```python
from build123d import *

# Parameters (mm, degrees)
SKETCH_1_R             = 120
EXTRUDE_1_DEPTH        = 20
SKETCH_2_R             = 100
EXTRUDE_2_DEPTH        = 50
SKETCH_3_R             = 8.5
CUT_EXTRUDE_1_DEPTH    = 80
SKETCH_4_R             = 20
EXTRUDE_3_DEPTH        = 20
HOLE_WIZARD_M161_D     = 14
HOLE_WIZARD_M161_DEPTH = 20
HOLE_WIZARD_M161_TIP   = 4.206024333
CHAMFER_1_SIZE         = 3
CHAMFER_2_SIZE         = 3


with BuildPart() as part:
    # Эскиз1 → Бобышка-Вытянуть1 (new body)
    with BuildSketch(Plane(origin=(0, 0, 0), x_dir=(1, 0, 0), z_dir=(0, 1, 0))):
        Circle(SKETCH_1_R)
    extrude(amount=EXTRUDE_1_DEPTH)

    # Эскиз2 → Бобышка-Вытянуть2 (add)
    with BuildSketch(Plane(origin=(0, 20, 0), x_dir=(1, 0, 0), z_dir=(0, 1, 0))):
        Circle(SKETCH_2_R)
    extrude(amount=EXTRUDE_2_DEPTH)

    # Эскиз3 → Вырез-Вытянуть1 (cut)
    with BuildSketch(Plane(origin=(0, 70, 0), x_dir=(1, 0, 0), z_dir=(0, 1, 0))):
        with Locations((0, 60)):
            Circle(SKETCH_3_R)
        with Locations((60, 0)):
            Circle(SKETCH_3_R)
        with Locations((0, -60)):
            Circle(SKETCH_3_R)
        with Locations((-60, 0)):
            Circle(SKETCH_3_R)
    extrude(amount=-CUT_EXTRUDE_1_DEPTH, mode=Mode.SUBTRACT)

    # Эскиз4 → Бобышка-Вытянуть3 (add)
    with BuildSketch(Plane.XZ):
        Circle(SKETCH_4_R)
    extrude(amount=EXTRUDE_3_DEPTH)

    # Отверстие обработанное метчиком M161
    with Locations(Plane(origin=(0, 70, 0), x_dir=(1, 0, 0), z_dir=(0, 1, 0))):
        with Locations((0, 0)):
            Hole(HOLE_WIZARD_M161_D / 2, depth=HOLE_WIZARD_M161_DEPTH)
            with Locations((0, 0, -(HOLE_WIZARD_M161_DEPTH + HOLE_WIZARD_M161_TIP / 2))):  # 118° drill point
                Cone(0, HOLE_WIZARD_M161_D / 2, HOLE_WIZARD_M161_TIP, mode=Mode.SUBTRACT)

    # Фаска1
    chamfer_1_edges = [part.edges().sort_by_distance(p)[0] for p in [
        (-120, 0, 0),
        (-120, 20, 0),
        (-100, 70, 0),
    ]]
    chamfer(chamfer_1_edges, length=CHAMFER_1_SIZE)

    # Фаска2
    chamfer_2_edges = [part.edges().sort_by_distance(p)[0] for p in [
        (-20, -20, 0),
    ]]
    chamfer(chamfer_2_edges, length=CHAMFER_2_SIZE)


solid = part.part
```
Source: CAD feature listing. Evaluate the final solid. Frame: model axes, mm. A direction names the side the tool comes from. Round coordinates to 2 decimals unless told otherwise and drop trailing zeros. Write each loop counter-clockwise with the first axis right and the second up, starting at its lowest first coordinate (ties: lowest second). Pieces come first, ordered by that corner, then holes. Notation, with made-up numbers: M 52,9.5 L 62,9.5 A17 ccw 62,27.5 Z; hole C -28,-36 d8. An arc over 180 degrees is marked long. Answer as a JSON object with one key per item and string values. Group by question number.
(1) Section query A-A on y = 7.5. Output: boundary loops of the cut face in (x, z), then the cut area to 3 significant figures.
(2) Reachability of faces 1 (the conical face through (108.213, 0.146, 44.867)), 2 (the flat face through (86, 20, -53)) from +Z, -Z, +X, -X, +Y, -Y: full face, straight path, thin tool, end or side. Return the list, or none.
(3) Mould query, pull axis X, two halves, no side actions, for faces 3 (the cylindrical face through (51.51, 35.49, -0.37)), 4 (the flat face through (-1, 70, 20)), 5 (the cylindrical face through (-4.336, -8.381, -19.524)). Classes: +X half, -X half, draft (parallel to the pull), parting line (faces both ways), or undercut.
(4) Section query B-B on y = -5.5. Output: boundary loops of the cut face in (x, z), then the cut area to 3 significant figures.
(5) Ray query, line 1 (X direction, y = 22, z = 0); line 2 (Z direction, x = 0, y = 56.5). Return the intervals inside material, ascending. Write a range as [from, to].
(6) First-contact query: pin 1 (4 mm diameter, centred on x = 92.5, y = 40.5, fed in from +Z); pin 2 (13.5 mm diameter, centred on x = -60, z = 0, fed in from -Y); pin 3 (12.5 mm diameter, centred on x = 0, z = 0, fed in from +Y); pin 4 (5 mm diameter, centred on y = 18, z = 61, fed in from -X). Flat tips, straight axial feed; report the tip coordinate or a pass-through.
Computed values:
{
 "1": {"outline": "C 0,0 d240; hole C -60,0 d17; hole C 0,-60 d17; hole C 0,60 d17; hole C 60,0 d17", "area": "44,300 mm^2"},
 "2": {"face 1": "-Y", "face 2": "+Y"},
 "3": {"face 3": "undercut", "face 4": "draft", "face 5": "parting line"},
 "4": {"outline": "C 0,0 d40", "area": "1,260 mm^2"},
 "5": {"line 1": "[-100, -68.5], [-51.5, 51.5], [68.5, 100]", "line 2": "[-100, -68.5], [-51.5, -7], [7, 51.5], [68.5, 100]"},
 "6": {"pin 1": "z = 42.54", "pin 2": "through", "pin 3": "y = 49.55", "pin 4": "x = -104.66"}
}
